CAD build for the part. Positions are in the model's coordinates, mm. Coordinates: 2 decimals unless noted, no trailing zeros. Order: outer loops, then holes, each group sorted by start corner. A loop starts at its lowest first (then second) coordinate and runs counter-clockwise, first axis right, second up. Notation, with made-up numbers: (14, 26.5) - (26, 26.5) arc R22 cw to (26, 45.5) - close; hole circle Ø8 at (33.25, -17). An arc over 180 degrees is marked (long way). Use one line per item in the form item = value.
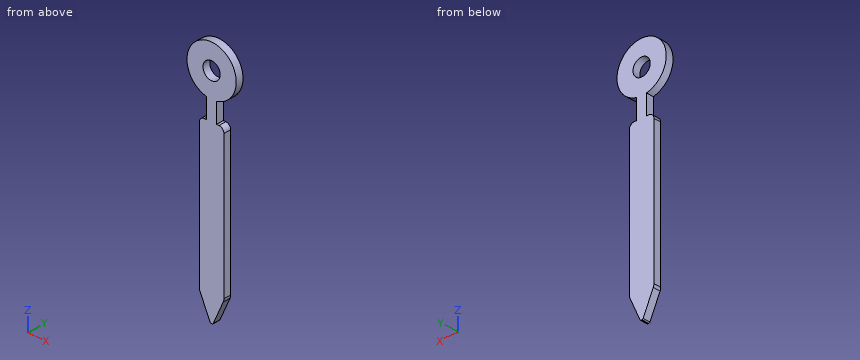
```python
from build123d import *

# Parameters (mm, degrees)
SKETCH1_R           = 0.35
BOSS_EXTRUDE1_DEPTH = 0.3


with BuildPart() as part:
    # Sketch1 → Boss-Extrude1 (new body)
    with BuildSketch(Plane(origin=(0, 0, 0), x_dir=(1, 0, 0), z_dir=(0, 1, 0))):
        with BuildLine():
            Line((0.063001459, 6.971107869), (0.473576452, 6.058718997))
            ThreePointArc((0.473576452, 6.058718997), (0.493319736, 5.998566184), (0.5, 5.935609593))
            Line((0.5, 5.935609593), (0.5, 0.2))
            ThreePointArc((0.5, 0.2), (0.441421356, 0.058578644), (0.3, 0))
            Line((0.3, 0), (0.2, 0))
            Line((0.2, 0), (0.2, -0.8))
            ThreePointArc((0.2, -0.8), (0, -2.779795897), (-0.2, -0.8))
            Line((-0.2, -0.8), (-0.2, 0))
            Line((-0.2, 0), (-0.3, 0))
            ThreePointArc((-0.3, 0), (-0.441421356, 0.058578644), (-0.5, 0.2))
            Line((-0.5, 0.2), (-0.5, 5.935609593))
            ThreePointArc((-0.5, 5.935609593), (-0.493319736, 5.998566184), (-0.473576452, 6.058718997))
            Line((-0.473576452, 6.058718997), (-0.063001459, 6.971107869))
            ThreePointArc((-0.063001459, 6.971107869), (-0.044922891, 6.992147816), (-0.018317305, 7))
            Line((-0.018317305, 7), (0.018317305, 7))
            ThreePointArc((0.018317305, 7), (0.044922891, 6.992147816), (0.063001459, 6.971107869))
        make_face()
        with Locations((0, -1.779795897)):
            Circle(SKETCH1_R, mode=Mode.SUBTRACT)
    extrude(amount=BOSS_EXTRUDE1_DEPTH)


solid = part.part
```
Item 1: Drill centre lines: line 1 (Z direction, x = 0, y = 0.15); line 2 (X direction, y = 0.25, z = -4.5); line 3 (X direction, y = 0.2, z = 0.5). Where is each one in solid material? Low to high. Write a range as [from, to].
Derived:
line_1 = [-7, 1.43], [2.13, 2.78]
line_2 = [-0.5, 0.5]
line_3 = [-0.2, 0.2]
Item 2: Cut at B-B, the plane z = -5.5. Write the cut outline in (x, y).
Derived:
outline = (-0.5, 0) - (0.5, 0) - (0.5, 0.3) - (-0.5, 0.3) - close
Item 3: Cut at A-A, the plane z = 2. Write the cut outline in (x, y), plus the area to 3 significant figures.
Derived:
outline = (-0.98, 0) - (-0.27, 0) - (-0.27, 0.3) - (-0.98, 0.3) - close; (0.27, 0) - (0.98, 0) - (0.98, 0.3) - (0.27, 0.3) - close
area = 0.422 mm²
